from build123d import *

# Parameters (mm, degrees)
BASE_FLANGE1_DEPTH  = 50.8
SKETCH8_R           = 12.7
CUT_EXTRUDE2_DEPTH  = 202.491653782
SKETCH9_R           = 25.36182522
BOSS_EXTRUDE1_DEPTH = 50.8


# Sheet-metal steps are written as plain solids
with BuildPart() as part:
    # Sketch2 → Base-Flange1 (new, symmetric)
    with BuildSketch(Plane.XY):
        with BuildLine():
            Line((38.1, 0), (38.1, 158.242))
            ThreePointArc((38.1, 158.242), (36.240128061, 162.732128061), (31.75, 164.592))
            Line((31.75, 164.592), (-31.75, 164.592))
            ThreePointArc((-31.75, 164.592), (-36.240128061, 162.732128061), (-38.1, 158.242))
            Line((-38.1, 158.242), (-38.1, 0))
            Line((-38.1, 0), (-45.72, 0))
            Line((-45.72, 0), (-45.72, 158.242))
            ThreePointArc((-45.72, 158.242), (-41.628281733, 168.120281733), (-31.75, 172.212))
            Line((-31.75, 172.212), (31.75, 172.212))
            ThreePointArc((31.75, 172.212), (41.628281733, 168.120281733), (45.72, 158.242))
            Line((45.72, 158.242), (45.72, 0))
            Line((45.72, 0), (38.1, 0))
        make_face()
    extrude(amount=BASE_FLANGE1_DEPTH, both=True)

    # Sketch8 → Cut-Extrude2 (cut, through all)
    with BuildSketch(Plane(origin=(45.72, 0, 0), x_dir=(0, 0, -1), z_dir=(1, 0, 0))):
        with BuildLine():
            Line((50.8, 0), (50.8, 158.242))
            Line((50.8, 158.242), (-2.510257588, 47.410018515))
            ThreePointArc((-2.510257588, 47.410018515), (-31.046261716, 33.655514771), (-50.8, 58.42))
            Line((-50.8, 58.42), (-50.8, 0))
            Line((-50.8, 0), (50.8, 0))
        make_face()
        with Locations((-25.4, 58.42)):
            Circle(SKETCH8_R)
    extrude(amount=-CUT_EXTRUDE2_DEPTH, mode=Mode.SUBTRACT)

    # Sketch9 → Boss-Extrude1 (add)
    with BuildSketch(Plane(origin=(0, 172.212, 0), x_dir=(1, 0, 0), z_dir=(0, 1, 0))):
        with Locations(Location((0, 0, 0), (0, 0, 270))):
            Circle(SKETCH9_R)
    extrude(amount=BOSS_EXTRUDE1_DEPTH)


solid = part.part
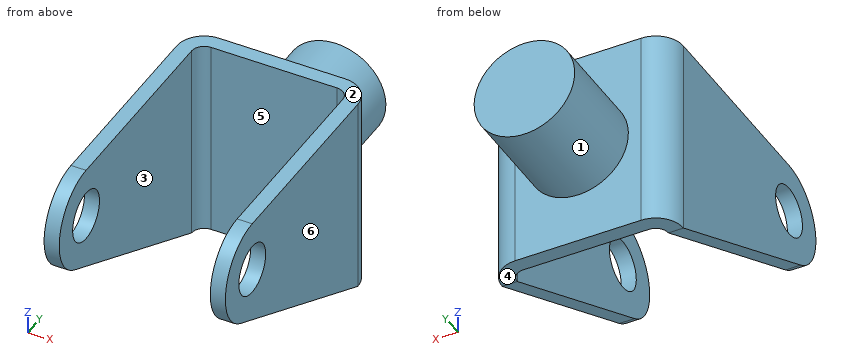
The model under review builds one solid part; all positions refer to its coordinate system, in mm. Face numbers are marked on the shaded views. A direction names the side the tool comes from. Give positions to 0.01 mm unless a question says otherwise; leave off trailing zeros. Write each loop counter-clockwise with the first axis right and the second up, starting at its lowest first coordinate (ties: lowest second). Pieces come first, ordered by that corner, then holes. Notation, with made-up numbers: M 87,-33.5 L 100,-33.5 A17 cw 100,-28.5 Z; hole C 1.5,22.25 d3. An arc over 180 degrees is marked long. One line per question, with ' | ' between items. Start each with the question number.
Item 1: Wall thickness on line 1 (X direction, y = 123, z = 36); line 2 (Y direction, x = -2, z = -25); line 3 (Y direction, x = 6, z = -27): over which ranges is each line inside the solid? List them lowest first. Write a range as from..to.
Item 2: We need section A-A on x = 0. Write out the cut boundary in (y, z), plus the area to 3 significant figures.
Item 3: Draft analysis for pull direction X (two halves, no side actions). For the marked faces 4, 5 and 6, state which applies: released by +X, released by -X, zero draft, split by the parting line, or undercut.
Item 4: We need section C-C on y = 52. Write out the cut boundary in (x, z), plus the area to 3 significant figures.
Item 5: For pin 1 (12 mm diameter, centred on x = -24.5, z = 38.5, fed in from +Y); pin 2 (23 mm diameter, centred on y = 58.42, z = 25.4, fed in from -X); pin 3 (4 mm diameter, centred on x = -34.5, z = 17.5, fed in from -Y); pin 4 (6 mm diameter, centred on x = 17.5, z = 28, fed in from -Y), all flat-tipped, find the tip position at first contact; note any pin that passes through.
Item 6: We need section D-D on z = 41. Write out the cut boundary in (x, y), plus the area to 3 significant figures.
Item 7: We need section B-B on z = 20.5. Write out the cut boundary in (x, y), plus the area to 3 significant figures.
Item 8: For the marked faces 1, 2 and 3, list the 3-axis set-ups (+Z, -Z, +X, -X, +Y, -Y) from which the entire face can be reached by the end or side of a thin tool; tool diameter is ignored.
Results found:
1) line 1: x = -45.72..-38.1, 38.1..45.72 | line 2: y = 164.59..223.01 | line 3: y = 164.59..172.21
2) outline: M 164.59,-50.8 L 172.21,-50.8 L 172.21,-25.36 L 223.01,-25.36 L 223.01,25.36 L 172.21,25.36 L 172.21,50.8 L 164.59,50.8 Z | area: 3,350 mm2
3) face 4: zero draft | face 5: undercut | face 6: released by +X
4) outline: M -45.72,0.3 L -38.1,0.3 L -38.1,14.44 L -45.72,14.44 Z; M -45.72,36.36 L -38.1,36.36 L -38.1,49.98 L -45.72,49.98 Z; M 38.1,0.3 L 45.72,0.3 L 45.72,14.44 L 38.1,14.44 Z; M 38.1,36.36 L 45.72,36.36 L 45.72,49.98 L 38.1,49.98 Z | area: 423 mm2
5) pin 1: stops at y = 172.21 | pin 2: passes through | pin 3: stops at y = 162.46 | pin 4: stops at y = 164.59
6) outline: M -45.72,38.38 L -38.1,38.38 L -38.1,158.24 A6.35 cw -31.75,164.59 L 31.75,164.59 A6.35 cw 38.1,158.24 L 38.1,38.38 L 45.72,38.38 L 45.72,158.24 A13.97 ccw 31.75,172.21 L -31.75,172.21 A13.97 ccw -45.72,158.24 Z | area: 2,550 mm2
7) outline: M -45.72,33.5 L -38.1,33.5 L -38.1,46.7 L -45.72,46.7 Z; M -45.72,70.14 L -38.1,70.14 L -38.1,158.24 A6.35 cw -31.75,164.59 L 31.75,164.59 A6.35 cw 38.1,158.24 L 38.1,70.14 L 45.72,70.14 L 45.72,158.24 A13.97 ccw 31.75,172.21 L 14.93,172.21 L 14.93,223.01 L -14.93,223.01 L -14.93,172.21 L -31.75,172.21 A13.97 ccw -45.72,158.24 Z; M 38.1,33.5 L 45.72,33.5 L 45.72,46.7 L 38.1,46.7 Z | area: 3,790 mm2
8) face 1: +Y | face 2: +Z, +X, -X, +Y, -Y | face 3: +Z, -Z, -Y
